```python
from build123d import *

# Parameters (mm, degrees)
EW_EXTRUDE_DEPTH = 30
FILLET1_R        = 1.5
FILLET2_R        = 1


with BuildPart() as part:
    # EW_SKETCH → EW_EXTRUDE (new body)
    with BuildSketch(Plane(origin=(0, 0, 0), x_dir=(0, 0, -1), z_dir=(1, 0, 0))):
        Polygon((0, 0), (4, 0), (4, 12.5), (-21.5, 12.5), (-21.5, -2.5), (-26, -2.5), (-26, -32.5), (-21.5, -32.5), (-21.5, -47.5), (4, -47.5), (4, -35), (0, -35), align=None)
    extrude(amount=EW_EXTRUDE_DEPTH)

    # fillet1
    fillet1_edges = [part.edges().sort_by_distance(p)[0] for p in [
        (15, -47.5, 21.5),
        (15, 12.5, 21.5),
    ]]
    fillet(fillet1_edges, radius=FILLET1_R)

    # fillet2
    fillet2_edges = [part.edges().sort_by_distance(p)[0] for p in [
        (15, -32.5, 26),
        (15, -2.5, 26),
    ]]
    fillet(fillet2_edges, radius=FILLET2_R)


solid = part.part
```
Part model, mm, in its own coordinate system. A direction names the side the tool comes from. Give positions to 0.01 mm unless a question says otherwise; leave off trailing zeros. Loops run counter-clockwise (first coordinate to the right, second up) from the corner with the lowest first, then second, coordinate; pieces in that order, holes last. Notation, with made-up numbers: M -1,28.5 L 21,28.5 A26 ccw 21,58.5 Z; hole C -5,54 d4. An arc over 180 degrees is marked long. Return JSON: item names as keys, results as strings.
1) Flat gauge pins, fed straight in: pin 1 Ø15 at (x, y) = (10, 7.5) entering from +Z; pin 2 Ø2 at (x, y) = (10.5, -19) entering from -Z; pin 3 Ø1 at (x, z) = (9.5, 22.5) entering from +Y; pin 4 Ø6 at (y, z) = (-31, 0) entering from -X. Where does each tip first touch, or does it go through?
Calculated:
{"pin 1": "stops at z = 21.5", "pin 2": "stops at z = 0", "pin 3": "stops at y = -2.5", "pin 4": "stops at x = 0"}
2) Drill centre lines: line 1 (Z direction, x = 6.5, y = -25.5); line 2 (Y direction, x = 7.5, z = 24.5); line 3 (Z direction, x = 17, y = -45). Where is each one in solid material? Low to high.
Calculated:
{"line 1": "z = 0 to 26", "line 2": "y = -32.5 to -2.5", "line 3": "z = -4 to 21.5"}
3) 3-axis set-ups, long thin cutter, end or side, ignore diameter. For faces 5 (the face through (15, 0, -2)), 6 (the face through (15, -17, 26)), 7 (the face through (15, -39, 21.5)): which of +Z, -Z, +X, -X, +Y, -Y reach the whole face in a straight line?
Calculated:
{"face 5": "-Z, +X, -X", "face 6": "+Z, +X, -X, +Y, -Y", "face 7": "+Z, +X, -X, -Y"}
4) Pull direction Y, two halves, no side cores. Call faces 1 (the face through (15, -35, -2)), 2 (the face through (15, 4, 21.5)), 3 (the face through (15, -2.5, 23)), 4 (the face through (15, -32.5, 23)): released by +Y, released by -Y, zero draft, split by the parting line, or undercut.
Calculated:
{"face 1": "undercut", "face 2": "zero draft", "face 3": "released by +Y", "face 4": "released by -Y"}
5) Saw through at B-B, the plane x = 13. List the corners of the cut face in (y, z).
Calculated:
{"outline": "M -47.5,-4 L -35,-4 L -35,0 L 0,0 L 0,-4 L 12.5,-4 L 12.5,20 A1.5 ccw 11,21.5 L -2.5,21.5 L -2.5,25 A1 ccw -3.5,26 L -31.5,26 A1 ccw -32.5,25 L -32.5,21.5 L -46,21.5 A1.5 ccw -47.5,20 Z"}
6) Saw through at A-A, the plane z = -1.5. List the corners of the cut face in (x, y).
Calculated:
{"outline": "M 0,-47.5 L 30,-47.5 L 30,-35 L 0,-35 Z; M 0,0 L 30,0 L 30,12.5 L 0,12.5 Z"}
7) Saw through at C-C, the plane y = -21. List the corners of the cut face in (x, z), then the cut area to 3 significant figures.
Calculated:
{"outline": "M 0,0 L 30,0 L 30,26 L 0,26 Z", "area": "780 mm2"}
8) Saw through at D-D, the plane y = -43.5. List the corners of the cut face in (x, z), then the cut area to 3 significant figures.
Calculated:
{"outline": "M 0,-4 L 30,-4 L 30,21.5 L 0,21.5 Z", "area": "765 mm2"}
